from build123d import *

# Parameters (mm, degrees)
SKETCH1_R           = 7.28
BOSS_EXTRUDE1_DEPTH = 20
FILLET1_R           = 2
SKETCH2_R           = 5
BOSS_EXTRUDE2_DEPTH = 15
SKETCH4_R           = 0.75
REVOLVE1_ANGLE      = 200


with BuildPart() as part:
    # Sketch1 → Boss-Extrude1 (new body)
    with BuildSketch(Plane.XY):
        Circle(SKETCH1_R)
    extrude(amount=BOSS_EXTRUDE1_DEPTH)

    # Fillet1
    fillet1_edges = [part.edges().sort_by_distance(p)[0] for p in [
        (-7.28, 0, 0),
        (-7.28, 0, 20),
    ]]
    fillet(fillet1_edges, radius=FILLET1_R)

    # Sketch2 → Boss-Extrude2 (add)
    with BuildSketch(Plane.XY.offset(20)):
        Circle(SKETCH2_R)
    extrude(amount=BOSS_EXTRUDE2_DEPTH)

    # Sketch4 → Revolve1 (revolve)
    with BuildSketch(Plane.XY.offset(35)):
        with Locations((0, 2.519535337)):
            Circle(SKETCH4_R)
    revolve(axis=Axis((-4.466449007, 0, 35), (1, 0, 0)), revolution_arc=REVOLVE1_ANGLE)


solid = part.part
Geometry check sheet. Reference: the model listing, model coordinates, mm. A direction names the side the tool comes from. Give positions to 0.01 mm unless a question says otherwise; leave off trailing zeros. Order: outer loops, then holes, each group sorted by start corner. A loop starts at its lowest first (then second) coordinate and runs counter-clockwise, first axis right, second up. Notation, with made-up numbers: (39, 85.5) - (45, 85.5) arc R31 cw to (45, 115.5) - close; hole circle Ø4 at (70.25, -37). An arc over 180 degrees is marked (long way). Use one line per item in the form item = value.
1) Access from +Z, -Z, +X, -X, +Y, -Y to the whole of each face (thin tool, end or side, straight path). Record for faces 1 (the face through (0, 0, 0)), 2 (the face through (-1.08, -4.88, 27.4)).
Working result:
face_1 = -Z, +X, -X, +Y, -Y
face_2 = +Z
2) Sectioned sample at B-B (x = 0). Record the boundary of the cut face in (y, z).
Working result:
outline = (-7.28, 2) arc R2 ccw to (-5.28, 0) - (5.28, 0) arc R2 ccw to (7.28, 2) - (7.28, 18) arc R2 ccw to (5.28, 20) - (5, 20) - (5, 35) - (3.27, 35) arc R3.27 ccw to (-3.27, 35) - (-5, 35) - (-5, 20) - (-5.28, 20) arc R2 ccw to (-7.28, 18) - close; hole (-1.77, 35) - (1.77, 35) arc R1.77 ccw to start
3) Material ranges on probe 1 along Z at (x, y) = (-3, 1); probe 2 along Y at (x, z) = (-6.5, 12); probe 3 along Z at (x, y) = (-4, -3.75), recorded low to high. Write a range as from..to.
Working result:
probe_1 = 0..35
probe_2 = -3.28..3.28
probe_3 = 0.01..19.99
4) Sectioned sample at C-C (z = 29). Record the boundary of the cut face in (x, y), and give its area (3 significant figures).
Working result:
outline = circle Ø10 at (0, 0)
area = 78.5 mm^2
5) Depth check by flat-ended pin: pin 1 Ø8 at (x, y) = (-1, -1) entering from +Z; pin 2 Ø6 at (x, z) = (4.5, 21.5) entering from +Y; pin 3 Ø1 at (x, z) = (-1, 28.5) entering from -Y; pin 4 Ø6 at (x, z) = (-4, 18.5) entering from -Y. Enter the tip coordinate at first touch or a pass-through.
Working result:
pin_1 = 38.27
pin_2 = 6.41
pin_3 = -4.97
pin_4 = -7.21
6) Sectioned sample at D-D (z = 11). Record the boundary of the cut face in (x, y).
Working result:
outline = circle Ø14.56 at (0, 0)
7) Sectioned sample at A-A (y = 0). Record the boundary of the cut face in (x, z), and give its area (3 significant figures).
Working result:
outline = (-7.28, 2) arc R2 ccw to (-5.28, 0) - (5.28, 0) arc R2 ccw to (7.28, 2) - (7.28, 18) arc R2 ccw to (5.28, 20) - (5, 20) - (5, 35) - (-5, 35) - (-5, 20) - (-5.28, 20) arc R2 ccw to (-7.28, 18) - close; circle Ø1.5 at (0, 37.52)
area = 440 mm^2
